from build123d import *

# Parameters (mm, degrees)
EXTRUDE_1_DEPTH     = 20
SKETCH_2_R          = 5
CUT_EXTRUDE_1_DEPTH = 232.102536476
SKETCH_3_W          = 32.604324085
SKETCH_3_H          = 2.91589364
SKETCH_3_W_2        = 9.316519648
SKETCH_3_H_2        = 2.560664992
SKETCH_3_W_3        = 11.683825265
EXTRUDE_2_DEPTH     = 48
SKETCH_5_R          = 5
CUT_EXTRUDE_2_DEPTH = 28


with BuildPart() as part:
    # 草图1 → 凸台-拉伸1 (new body)
    with BuildSketch(Plane.XY):
        Polygon((17.319300214, 114.65132411), (167.319300214, 114.65132411), (199.6583488, -20.002569933), (-21.915099237, -20.002569933), align=None)
    extrude(amount=EXTRUDE_1_DEPTH)

    # 草图2 → 切除-拉伸1 (cut, through all)
    with BuildSketch(Plane.XY.offset(20)):
        with Locations((77.319300214, 84.433001075)):
            Circle(SKETCH_2_R)
        with Locations((76.069300214, 34.448628517)):
            Circle(SKETCH_2_R)
        with Locations(Location((108.569300214, 34.448628517, 0), (0, 0, 180))):
            Circle(SKETCH_2_R)
        with Locations(Location((107.319300214, 84.433001075, 0), (0, 0, 180))):
            Circle(SKETCH_2_R)
    extrude(amount=-CUT_EXTRUDE_1_DEPTH, mode=Mode.SUBTRACT)

    # 草图3 → 凸台-拉伸2 (add)
    with BuildSketch(Plane.XY.offset(20)):
        with Locations((76.385027523, -13.259318303)):
            Rectangle(SKETCH_3_W, SKETCH_3_H)
        with Locations((67.171853972, 82.139796752)):
            Rectangle(SKETCH_3_W_2, SKETCH_3_H_2)
        with Locations((88.67813561, 82.139796752)):
            Rectangle(SKETCH_3_W_3, SKETCH_3_H_2)
    extrude(amount=-EXTRUDE_2_DEPTH)

    # 草图5 → 切除-拉伸2 (cut)
    with BuildSketch(Plane(origin=(0, 0, 0), x_dir=(-1, 0, 0), z_dir=(0, 0, -1))):
        with Locations((-156.886362857, -0.002569933)):
            Circle(SKETCH_5_R)
        with Locations((-12.853580473, -0.002569933)):
            Circle(SKETCH_5_R)
    extrude(amount=-CUT_EXTRUDE_2_DEPTH, mode=Mode.SUBTRACT)


solid = part.part
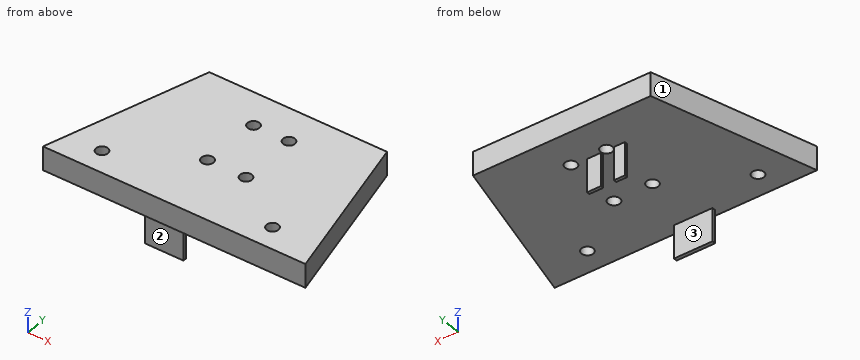
The listing builds one solid part. Answer for the finished solid, in the listing's coordinates (mm). Face numbers are marked on the shaded views. A direction names the side the tool comes from. Give positions to 0.01 mm unless a question says otherwise; leave off trailing zeros. Write each loop counter-clockwise with the first axis right and the second up, starting at its lowest first coordinate (ties: lowest second). Pieces come first, ordered by that corner, then holes. Notation, with made-up numbers: (-38, -36) - (8, -36) arc R23 ccw to (8, 1) - close; hole circle Ø7 at (-38.5, 42). An arc over 180 degrees is marked (long way). One line per question, with ' | ' between items. Start each with the question number.
1. Section A-A, the plane z = -18 is taken. Determine the outline of the cut face in (x, y).
2. Straight lines are drawn through the part: line 1 (X direction, y = 2.5, z = 9.5) (3 decimals); line 2 (Z direction, x = 90.5, y = 10); line 3 (Y direction, x = 75.5, z = 0.5). For each, find the intervals that lie inside material, in ascending order.
3. Section C-C, the plane z = 16 is taken. Determine the outline of the cut face in (x, y).
4. Section B-B, the plane x = 14 is taken. Determine the outline of the cut face in (y, z), then the cut area to 3 significant figures.
5. Given P1, Ø22.5, axis at x = 83.5, z = -11.5, coming from the -Y side; P2, Ø1.3, axis at y = 82, z = -15.5, coming from the -X side; P3, Ø10, axis at x = 90, y = 32, coming from the -Z side, each flat-ended and moving along its own axis, determine where each tip first touches the part or whether it passes through.
6. Section D-D, the plane y = 45.5 is taken. Determine the outline of the cut face in (x, z), then the cut area to 3 significant figures.
7. For the marked faces 1, 2 and 3, determine the directions among +Z, -Z, +X, -X, +Y, -Y from which every point of the face is accessible in a straight line to the end or side of a thin tool.
Result:
1) outline: (60.08, -14.72) - (92.69, -14.72) - (92.69, -11.8) - (60.08, -11.8) - close; (62.51, 80.86) - (71.83, 80.86) - (71.83, 83.42) - (62.51, 83.42) - close; (82.84, 80.86) - (94.52, 80.86) - (94.52, 83.42) - (82.84, 83.42) - close
2) line 1: x = -15.358 to 8.525, 17.182 to 152.558, 161.215 to 194.254 | line 2: z = 0 to 20 | line 3: y = -20 to 29.48, 39.42 to 79.78, 89.09 to 114.65
3) outline: (-21.92, -20) - (199.66, -20) - (167.32, 114.65) - (17.32, 114.65) - close; hole circle Ø10 at (12.85, 0); hole circle Ø10 at (76.07, 34.45); hole circle Ø10 at (77.32, 84.43); hole circle Ø10 at (107.32, 84.43); hole circle Ø10 at (108.57, 34.45); hole circle Ø10 at (156.89, 0)
4) outline: (-20, 0) - (-4.87, 0) - (-4.87, 20) - (-20, 20) - close; (4.86, 0) - (103.26, 0) - (103.26, 20) - (4.86, 20) - close | area: 2,270 mm2
5) P1: stops at y = -14.72 | P2: stops at x = 62.51 | P3: stops at z = 0
6) outline: (-2.83, 0) - (183.93, 0) - (183.93, 20) - (-2.83, 20) - close | area: 3,740 mm2
7) face 1: +Z, -Z, -X, +Y | face 2: -Z, +X, -X, -Y | face 3: -Z, +X, -X
